Part model, mm, in its own coordinate system. Face numbers are marked on the shaded views. A direction names the side the tool comes from. Round coordinates to 2 decimals unless told otherwise and drop trailing zeros. Loops run counter-clockwise (first coordinate to the right, second up) from the corner with the lowest first, then second, coordinate; pieces in that order, holes last. Notation, with made-up numbers: (-40, -16) -> (17, -16) arc R13 cw to (17, 4) -> close; hole circle Ø4 at (10.5, 51.25). An arc over 180 degrees is marked (long way). Answer as a JSON object with one key per item and string values. Group by question number.
Solid Edge part; units mm, degrees
sketch "Sketch1" plane through (0, 0, 0) normal (0, -1, 0) x (1, 0, 0)
  line L0 (15, 50) -> (25, 50)
  line L1 (25, 50) -> (40, 30)
  line L2 (40, 30) -> (55, 50)
  line L3 (65, 50) -> (55, 50)
  line L4 (65, 10) -> (65, 50)
  line L5 (80, 10) -> (65, 10)
  line L6 (80, 0) -> (80, 10)
  line L7 (60, 0) -> (80, 0)
  line L8 (60, 5) -> (60, 0)
  line L9 (20, 5) -> (60, 5)
  line L10 (20, 0) -> (20, 5)
  line L11 (0, 0) -> (20, 0)
  line L12 (0, 0) -> (0, 10)
  line L13 (0, 10) -> (15, 10)
  line L14 (15, 10) -> (15, 50)
extrude "Protrusion1" add sketch "Sketch1" against normal blind 40
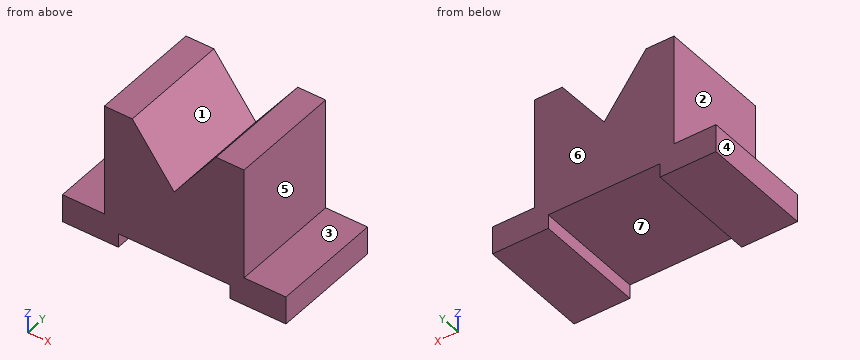
Item 1: Band-saw the part on D-D, the plane z = 33.5. List the corners of the cut face in (x, y) (3 decimals).
Item 2: Which spindle directions (+Z, -Z, +X, -X, +Y, -Y) get a long thin tool onto all of the face, cutting with end or side? Do the marked faces 1, 2 and 3. Say none if no direction does.
Item 3: Band-saw the part on C-C, the plane x = 38.5. List the corners of the cut face in (y, z), plus the area to 3 significant figures.
Item 4: Band-saw the part on A-A, the plane z = 4. List the corners of the cut face in (x, y), plus the area to 3 significant figures.
Item 5: Drop flat-ended pins along their axis: pin 1 Ø20 at (y, z) = (25.5, 27) entering from +X; pin 2 Ø20 at (y, z) = (23.5, 23.5) entering from -X; pin 3 Ø3 at (x, y) = (30.5, 6) entering from +Z. Give the stop position or say it passes through.
Item 6: Drill centre lines: line 1 (X direction, y = 9, z = 19); line 2 (Z direction, x = 20.5, y = 12); line 3 (X direction, y = 5, z = 40.5) (3 decimals). Where is each one in solid material? Low to high.
Item 7: Band-saw the part on B-B, the plane y = 16.5. List the corners of the cut face in (x, z).
Item 8: Two-plate mould, pull along X, no slides. Class the marked faces 4, 5, 6 and 7: pulls with the +X half, pulls with the -X half, needs draft (parallel to the pull), parting line crosses it, or undercut.
Entries:
{
 "1": {"outline": "(15, 0) -> (37.375, 0) -> (37.375, 40) -> (15, 40) -> close; (42.625, 0) -> (65, 0) -> (65, 40) -> (42.625, 40) -> close"},
 "2": {"face 1": "+Z, +Y, -Y", "face 2": "+Z, -X, +Y, -Y", "face 3": "+Z, +X, +Y, -Y"},
 "3": {"outline": "(0, 5) -> (40, 5) -> (40, 32) -> (0, 32) -> close", "area": "1,080 mm²"},
 "4": {"outline": "(0, 0) -> (20, 0) -> (20, 40) -> (0, 40) -> close; (60, 0) -> (80, 0) -> (80, 40) -> (60, 40) -> close", "area": "1,600 mm²"},
 "5": {"pin 1": "x = 65", "pin 2": "x = 15", "pin 3": "z = 44.67"},
 "6": {"line 1": "15 to 65", "line 2": "5 to 50", "line 3": "15 to 32.125, 47.875 to 65"},
 "7": {"outline": "(0, 0) -> (20, 0) -> (20, 5) -> (60, 5) -> (60, 0) -> (80, 0) -> (80, 10) -> (65, 10) -> (65, 50) -> (55, 50) -> (40, 30) -> (25, 50) -> (15, 50) -> (15, 10) -> (0, 10) -> close"},
 "8": {"face 4": "pulls with the -X half", "face 5": "pulls with the +X half", "face 6": "needs draft", "face 7": "undercut"}
}
